Autodesk Inventor part; units mm, degrees
ref_plane "YZ Plane" through (0, 0, 0) normal (1, 0, 0) x (0, 1, 0)
ref_plane "XZ Plane" through (0, 0, 0) normal (0, 1, 0) x (-1, 0, 0)
ref_plane "XY Plane" through (0, 0, 0) normal (0, 0, 1) x (1, 0, 0)
sketch "Boceto1" plane through (0, 0, 0) normal (0, 1, 0) x (-1, 0, 0)
  point P0 (0, 0)
sketch "Boceto2" plane through (0, 0, 0) normal (0, 1, 0) x (-1, 0, 0)
  line L0 (0, 0) -> (-30, 0)
  line L1 (-30, 0) -> (-30, -90)
  line L2 (-30, -90) -> (0, -90)
  line L3 (0, -90) -> (0, 0)
  dimension "d0" = 30
  dimension "d1" = 90
extrude "Extrusión1" add sketch "Boceto2" along normal blind 5
sketch "Boceto3" plane through (0, 0, 0) normal (0, 0, 1) x (1, 0, 0)
  circle A0 centre (25, 2.5) radius 1.5
  circle A1 centre (5, 2.5) radius 1.5
  line L0 (0, 0) -> (0, 5)
  line L1 (30, 0) -> (30, 5)
  line L2 (0, 0) -> (30, 0)
  dimension "d4" = 3
  dimension "d5" = 3
  dimension "d6" = 5
  dimension "d7" = 5
  dimension "d8" = 2.5
  dimension "d9" = 2.5
extrude "Extrusión2" cut sketch "Boceto3" against normal blind 3
sketch "Boceto4" plane through (30, 0, -90) normal (0, 0, -1) x (-1, 0, 0)
  circle A0 centre (5, 2.5) radius 1.5
  circle A1 centre (5, 2.5) radius 1.5
  circle A2 centre (25, 2.5) radius 1.5
  circle A3 centre (25, 2.5) radius 1.5
  point P0 (30, 0)
extrude "Extrusión3" cut sketch "Boceto4" against normal blind 3
properties part number "Interno"
The listing builds one solid part. Answer for the finished solid, in the listing's coordinates (mm). A direction names the side the tool comes from. Coordinates: 2 decimals unless noted, no trailing zeros. Write each loop counter-clockwise with the first axis right and the second up, starting at its lowest first coordinate (ties: lowest second). Pieces come first, ordered by that corner, then holes. Notation, with made-up numbers: M 84.5,72.5 L 97.5,72.5 A31 cw 97.5,103.5 Z; hole C 39,4 d2. An arc over 180 degrees is marked long. Put each result on its own line as item: value. Start each with the question number.
1. A flat-ended cylindrical pin translates along its axis: P1, Ø2.5, axis at x = 5, y = 2.5, coming from the +Z side. Find the tip coordinate at first contact, or state that the pin passes through.
2. Consider line 1 (Y direction, x = 5, z = -2); line 2 (Z direction, x = 24.5, y = 2.55). Determine where each line is inside the solid, lowest interval first. Write a range as from..to.
3. Which of the six approach directions +Z, -Z, +X, -X, +Y, -Y give full straight-line access (tool end or side, diameter ignored) to faces 4 (the flat face through (30, 2, -44)), 5 (the flat face through (5, 3, -3)), 6 (the cylindrical face through (6.2, 1.6, -88.5))?
4. For a pull along Y with two mould halves and no side action, classify faces 1 (the flat face through (0, 2, -46)), 2 (the cylindrical face through (26.5, 2.57, -88.52)), 3 (the flat face through (15, 0, -44)) as pulls with the +Y half, pulls with the -Y half, needs draft (parallel to the pull), parting line crosses it, or undercut.
5. A cutting plane is placed at A-A on x = 25. Write down the section's boundary in (y, z), then the cut area to 3 significant figures.
Resolved:
1. P1: stops at z = -3
2. line 1: y = 0..1, 4..5
2. line 2: z = -87..-3
3. face 4: +Z, -Z, +X, +Y, -Y
3. face 5: +Z
3. face 6: -Z
4. face 1: needs draft
4. face 2: undercut
4. face 3: pulls with the -Y half
5. outline: M 0,-90 L 1,-90 L 1,-87 L 4,-87 L 4,-90 L 5,-90 L 5,0 L 4,0 L 4,-3 L 1,-3 L 1,0 L 0,0 Z
5. area: 432 mm2
